The drawing under review shows one solid part. Ordinate dimensions are in mm from its lowest x, y, z. A direction names the side the tool comes from. Give positions to 0.01 mm unless a question says otherwise; leave off trailing zeros. Write each loop counter-clockwise with the first axis right and the second up, starting at its lowest first coordinate (ties: lowest second). Pieces come first, ordered by that corner, then holes.
Q1. For line 1 (X direction, y = 70.5, z = 48); line 2 (Y direction, x = 67, z = 49.5), list the stretches that pass through material, from the lowest coordinate up.
Q2. We need section A-A (z = 35.5). Write out the cut boundary in (x, y).
Q3. Mouldability with a two-part tool opening along Z and no side actions: class the marked faces 1, 2 and 3 as released by +Z, released by -Z, zero draft, split by the parting line, or undercut.
Q4. Machinability: for the marked faces 4 and 5, which of the approach directions +Z, -Z, +X, -X, +Y, -Y give a long, thin tool a straight path to every point of the face, cutting with its end or side? Answer none if there is none.
Q5. Insertion check: P1, Ø4, axis at x = 31.5, y = 61, coming from the -Z side; P2, Ø12, axis at y = 77.5, z = 30, coming from the +X side; P3, Ø9.5, axis at x = 68, z = 26.5, coming from the +Y side. Each pin has a flat end and moves straight along its axis. Give the tip position at first contact, or say it passes through.
Q6. We need section B-B (y = 83.5). Write out the cut boundary in (x, z), then the cut area to 3 significant figures.
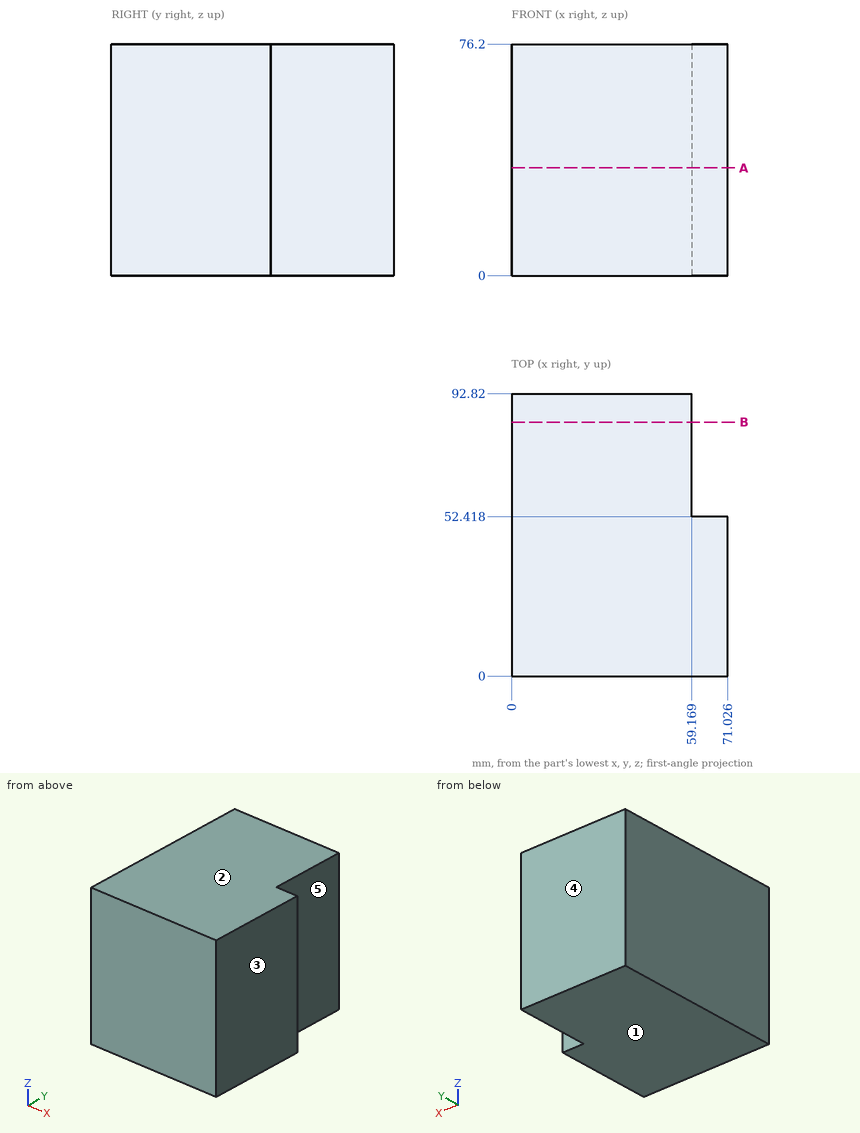
Computed:
1. line 1: x = 0 to 59.17
1. line 2: y = 0 to 52.42
2. outline: (0, 0) - (71.03, 0) - (71.03, 52.42) - (59.17, 52.42) - (59.17, 92.82) - (0, 92.82) - close
3. face 1: released by -Z
3. face 2: released by +Z
3. face 3: zero draft
4. face 4: +Z, -Z, +X, -X, +Y
4. face 5: +Z, -Z, +X, +Y
5. P1: stops at z = 0
5. P2: stops at x = 59.17
5. P3: stops at y = 52.42
6. outline: (0, 0) - (59.17, 0) - (59.17, 76.2) - (0, 76.2) - close
6. area: 4,510 mm2
